```python
from build123d import *

# Parameters (mm, degrees)
SKETCH1_R           = 1.6
BOSS_EXTRUDE1_DEPTH = 3
SKETCH2_R           = 10
CUT_EXTRUDE1_DEPTH  = 178.200787705
BOSS_EXTRUDE2_DEPTH = 3
SKETCH4_R           = 1.6
CUT_EXTRUDE2_DEPTH  = 10
SKETCH5_R           = 1.6
CUT_EXTRUDE4_DEPTH  = 233.870824119
SKETCH6_R           = 1.6
CUT_EXTRUDE5_DEPTH  = 233.870824119


with BuildPart() as part:
    # Sketch1 → Boss-Extrude1 (new body)
    with BuildSketch(Plane.XY):
        Polygon((-65.110127969, 48.691011888), (-135.939165656, -73.988480037), (-113.05241431, -113.629496188), (28.605661063, -113.629496188), (51.492412409, -73.988480037), (-19.336625277, 48.691011888), align=None)
        with Locations((-15.850309664, -7.988480037)):
            Circle(SKETCH1_R, mode=Mode.SUBTRACT)
        with Locations((4.149690336, -42.629496188)):
            Circle(SKETCH1_R, mode=Mode.SUBTRACT)
        with Locations((-80.472087929, -36.060276806)):
            Circle(SKETCH1_R, mode=Mode.SUBTRACT)
        with Locations((-52.472087929, -84.557699418)):
            Circle(SKETCH1_R, mode=Mode.SUBTRACT)
        with BuildLine():
            Line((-42.223376623, -10.308988112), (-2.819220751, -14.058988112))
            ThreePointArc((-2.819220751, -14.058988112), (5.624526936, -18.933988112), (5.624526936, -28.683988112))
            Line((5.624526936, -28.683988112), (-10.829955736, -64.683988112))
            ThreePointArc((-10.829955736, -64.683988112), (-73.616797511, -64.683988112), (-42.223376623, -10.308988112))
        make_face(mode=Mode.SUBTRACT)
    extrude(amount=BOSS_EXTRUDE1_DEPTH)

    # Sketch2 → Cut-Extrude1 (cut, through all)
    with BuildSketch(Plane.XY.offset(3)):
        with Locations((-2.819220751, -23.808988112)):
            Circle(SKETCH2_R)
    extrude(amount=-CUT_EXTRUDE1_DEPTH, mode=Mode.SUBTRACT)

    # Sketch3 → Boss-Extrude2 (add)
    with BuildSketch(Plane.XY.offset(3)):
        with BuildLine():
            ThreePointArc((78.022043807, -46.558988112), (34.284577527, 46.206814241), (-65.110127969, 71.488281011))
            ThreePointArc((-65.110127969, 71.488281011), (-118.731330774, -139.324790466), (78.022043807, -46.558988112))
        make_face()
        Polygon((-135.939165656, -73.988480037), (-65.110127969, 48.691011888), (-19.336625277, 48.691011888), (51.492412409, -73.988480037), (28.605661063, -113.629496188), (-113.05241431, -113.629496188), align=None, mode=Mode.SUBTRACT)
    extrude(amount=-BOSS_EXTRUDE2_DEPTH)

    # Sketch4 → Cut-Extrude2 (cut)
    with BuildSketch(Plane(origin=(0, 0, 0), x_dir=(-1, 0, 0), z_dir=(0, 0, -1))):
        with Locations((-15.389294768, -99.586461705)):
            Circle(SKETCH4_R)
        with Locations((-17.802637284, -127.171092895)):
            Circle(SKETCH4_R)
        with Locations((86.467923808, -145.829873387)):
            Circle(SKETCH4_R)
        with Locations((64.041857466, 16.578685607)):
            Circle(SKETCH4_R)
        with Locations((97.309290774, -30.932132962)):
            Circle(SKETCH4_R)
        with Locations((104.180307636, 44.683930988)):
            Circle(SKETCH4_R)
        with Locations((137.447740944, -2.82688758)):
            Circle(SKETCH4_R)
        with Locations((90.232180337, -102.804224376)):
            Circle(SKETCH4_R)
    extrude(amount=-CUT_EXTRUDE2_DEPTH, mode=Mode.SUBTRACT)

    # Sketch5 → Cut-Extrude4 (cut, through all)
    with BuildSketch(Plane(origin=(0, 0, 0), x_dir=(-1, 0, 0), z_dir=(0, 0, -1))):
        with Locations((82.277051548, -69.683988112)):
            Circle(SKETCH5_R)
        with Locations((134.238575775, -99.683988112)):
            Circle(SKETCH5_R)
        with Locations((96.585864973, -77.945185395)):
            Circle(SKETCH5_R)
        Polygon((82.277051548, -69.683988112), (83.077051548, -68.298347466), (97.385864973, -76.559544749), (96.585864973, -77.945185395), (95.785864973, -79.330826041), (81.497868277, -71.081440591), align=None)
    extrude(amount=-CUT_EXTRUDE4_DEPTH, mode=Mode.SUBTRACT)

    # Sketch6 → Cut-Extrude5 (cut, through all)
    with BuildSketch(Plane(origin=(0, 0, 0), x_dir=(-1, 0, 0), z_dir=(0, 0, -1))):
        with Locations((155.831472002, -46.59864482)):
            Circle(SKETCH6_R)
        with Locations((151.955243084, -75.982080937)):
            Circle(SKETCH6_R)
        with Locations((125.615678054, -68.919488348)):
            Circle(SKETCH6_R)
        with Locations((103.284288585, -107.598589514)):
            Circle(SKETCH6_R)
        with Locations((122.570455698, -126.878025659)):
            Circle(SKETCH6_R)
        with Locations((99.061768029, -144.926656432)):
            Circle(SKETCH6_R)
        with Locations((98.993080596, 51.848336915)):
            Circle(SKETCH6_R)
        with Locations(Location((71.608164009, 63.183142259, 0), (0, 0, 180))):
            Circle(SKETCH6_R)
        with Locations((64.554766093, 36.841113525)):
            Circle(SKETCH6_R)
        with Locations((12.838589238, 63.183142259)):
            Circle(SKETCH6_R)
        with Locations((-14.546327349, 51.848336915)):
            Circle(SKETCH6_R)
        with Locations((19.891987154, 36.841113525)):
            Circle(SKETCH6_R)
        with Locations((-41.168924808, -68.919488348)):
            Circle(SKETCH6_R)
        with Locations((-67.508489837, -75.982080937)):
            Circle(SKETCH6_R)
        with Locations((-71.384718755, -46.59864482)):
            Circle(SKETCH6_R)
        with Locations((-38.123702451, -126.878025659)):
            Circle(SKETCH6_R)
        with Locations((-14.615014783, -144.926656432)):
            Circle(SKETCH6_R)
        with Locations((-18.837535338, -107.598589514)):
            Circle(SKETCH6_R)
    extrude(amount=-CUT_EXTRUDE5_DEPTH, mode=Mode.SUBTRACT)


solid = part.part
```
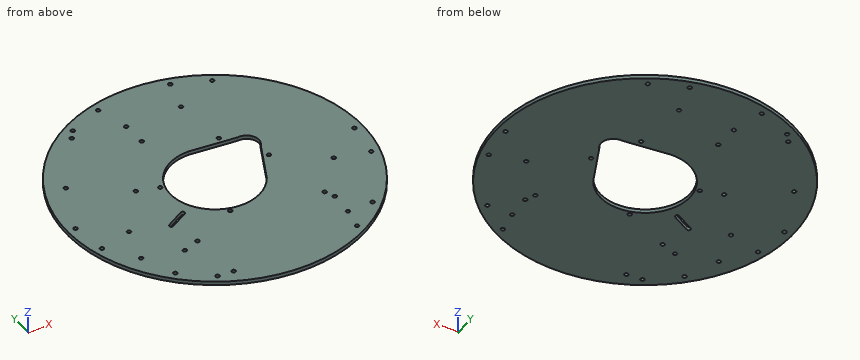
Geometry check sheet. Reference: the model listing, model coordinates, mm. Round coordinates to 2 decimals unless told otherwise and drop trailing zeros. Order: outer loops, then holes, each group sorted by start corner. A loop starts at its lowest first (then second) coordinate and runs counter-clockwise, first axis right, second up. Notation, with made-up numbers: (35.5, -38.75) - (75.5, -38.75) arc R14 ccw to (75.5, -26.75) - close; hole circle Ø11 at (76, 47). An arc over 180 degrees is marked (long way). Use a Markdown table: item, result. Add a question column.
(1) Depth check by flat-ended pin: pin 1 (4 mm diameter, centred on x = -151.96, y = -75.98, fed in from -Z); pin 2 (2.5 mm diameter, centred on x = -52.47, y = -84.56, fed in from -Z); pin 3 (1 mm diameter, centred on x = -93, z = 1, fed in from -Y). Enter the tip coordinate at first touch or a pass-through.
(2) Sectioned sample at D-D, the plane x = 26. Enter the section's corners in (y, z).
(3) Sectioned sample at A-A, the plane x = -58. Enter the section's corners in (y, z).
(4) Sectioned sample at B-B, the plane y = -115.5. Enter the section's corners in (x, z), and give its area (3 significant figures).
(5) Material ranges on line 1 along X through (y, z) = (-126, 2.9); line 2 along X through (y, z) = (-101, 1.9); line 3 along Y through (x, z) = (-85, 2.15), recorded low to high. Write a range as [from, to].
(6) Sectioned sample at C-C, the plane z = 2.45. Count the separate pieces of the cut face and the enclosed holes in it, and give its area (3 significant figures).
Answers below:
| question | item | result |
|---|---|---|
| 1 | pin 1 | z = 0 |
| 1 | pin 2 | through |
| 1 | pin 3 | y = -155.79 |
| 2 | outline | (-145.58, 0) - (52.46, 0) - (52.46, 3) - (-145.58, 3) - close |
| 3 | outline | (-165.76, 0) - (-79.2, 0) - (-79.2, 3) - (-165.76, 3) - close; (-13.92, 0) - (72.65, 0) - (72.65, 3) - (-13.92, 3) - close |
| 4 | outline | (-140.74, 0) - (56.3, 0) - (56.3, 3) - (-140.74, 3) - close |
| 4 | area | 591 mm² |
| 5 | line 1 | [-132.49, -123.91], [-121.23, 16.71], [18.89, 36.79], [39.46, 48.04] |
| 5 | line 2 | [-149.44, -135.15], [-133.33, 14.64], [16.14, 64.99] |
| 5 | line 3 | [-158.94, -146.47], [-145.19, -73.1], [-69.41, 65.82] |
| 6 | separate pieces | 1 |
| 6 | enclosed holes | 33 |
| 6 | area | 40,400 mm² |
